from build123d import *

# Parameters (mm, degrees)
F0_R     = 10.8555352801
F1_DEPTH = 13
F2_T     = -2.5
F3_R     = 3.906627993
F4_DEPTH = 11.4
F5_T     = -1
F6_W     = 5.8806912699
F6_H     = 0.9425205584
F7_DEPTH = 12.4


with BuildPart() as f1:
    # F0 (on Top) → F1 (new body)
    with BuildSketch(Plane.XY):
        Circle(F0_R)
    extrude(amount=F1_DEPTH)

    # F2
    f2_openings = [f1.faces().sort_by_distance(p)[0] for p in [
        (0, 0, 0),
    ]]
    offset(amount=F2_T, openings=f2_openings)

    # F3 (on face) → F4 (join)
    with BuildSketch(Plane.XY.offset(13)):
        Circle(F3_R)
    extrude(amount=F4_DEPTH)

    # F5
    f5_openings = [f1.faces().sort_by_distance(p)[0] for p in [
        (0, 0, 24.4),
    ]]
    offset(amount=F5_T, openings=f5_openings, kind=Kind.INTERSECTION)

    # F6 (on face) → F7 (join)
    with BuildSketch(Plane.XY.offset(24.4)):
        with Locations((0.0686239588, 2.1773161103)):
            Rectangle(F6_W, F6_H)
    extrude(amount=-F7_DEPTH)


solid = f1.part
Check sheet for the modelled part. Datum: model origin and axes. Units: mm. A direction names the side the tool comes from. Coordinates: 2 decimals unless noted, no trailing zeros. Loops run counter-clockwise (first coordinate to the right, second up) from the corner with the lowest first, then second, coordinate; pieces in that order, holes last. Notation, with made-up numbers: (45, 48.25) -> (83, 48.25) arc R22 cw to (83, 73.25) -> close; hole circle Ø10 at (-13, 75.25). An arc over 180 degrees is marked (long way). Answer in a Markdown table with one row per item.
1. Sectioned sample at D-D, the plane y = -5. Record the boundary of the cut face in (x, z), then the cut area to 3 significant figures.
Check values:
| item | result |
|---|---|
| outline | (-9.64, 0) -> (-6.69, 0) -> (-6.69, 10.5) -> (6.69, 10.5) -> (6.69, 0) -> (9.64, 0) -> (9.64, 13) -> (-9.64, 13) -> close; hole (-8.49, 1) -> (-7.91, 1) -> (-7.91, 11.5) -> (7.91, 11.5) -> (7.91, 1) -> (8.49, 1) -> (8.49, 12) -> (-8.49, 12) -> close |
| area | 89.1 mm2 |
2. Sectioned sample at B-B, the plane x = 0. Record the boundary of the cut face in (y, z).
Check values:
| item | result |
|---|---|
| outline | (-10.86, 0) -> (-8.36, 0) -> (-8.36, 10.5) -> (8.36, 10.5) -> (8.36, 0) -> (10.86, 0) -> (10.86, 13) -> (3.91, 13) -> (3.91, 24.4) -> (2.91, 24.4) -> (2.91, 12) -> (9.86, 12) -> (9.86, 1) -> (9.36, 1) -> (9.36, 11.5) -> (-9.36, 11.5) -> (-9.36, 1) -> (-9.86, 1) -> (-9.86, 12) -> (-2.91, 12) -> (-2.91, 24.4) -> (-3.91, 24.4) -> (-3.91, 13) -> (-10.86, 13) -> close; (1.71, 12) -> (2.65, 12) -> (2.65, 24.4) -> (1.71, 24.4) -> close |
3. Material ranges on line 1 along Y through (x, z) = (0, 9.25); line 2 along Z through (x, y) = (0.25, 2); line 3 along Z through (x, y) = (-5, -8), recorded low to high. Write a range as [from, to].
Check values:
| item | result |
|---|---|
| line 1 | y = [-10.86, -9.86], [-9.36, -8.36], [8.36, 9.36], [9.86, 10.86] |
| line 2 | z = [10.5, 11.5], [12, 24.4] |
| line 3 | z = [0, 1], [12, 13] |
4. Release check for a two-part mould opening along Y. For faces 1 (the face through (0, 2, 24.4)), 2 (the face through (10.354, 3.261, 6.409)), 3 (the face through (0, 2, 12)) record: released by +Y, released by -Y, zero draft, split by the parting line, or undercut.
Check values:
| item | result |
|---|---|
| face 1 | zero draft |
| face 2 | split by the parting line |
| face 3 | undercut |
5. Go/stop test with flat-tipped pins: pin 1 (3 mm diameter, centred on y = 1.5, z = 13.5, fed in from +X); pin 2 (8.5 mm diameter, centred on x = 2.5, y = -2, fed in from -Z); pin 3 (8 mm diameter, centred on x = -8, z = 11.5, fed in from -Y); pin 4 (1.5 mm diameter, centred on x = -1, z = 6, fed in from +Y). Record where each tip stops, or that it passes through.
Check values:
| item | result |
|---|---|
| pin 1 | stops at x = 10.86 |
| pin 2 | stops at z = 10.5 |
| pin 3 | stops at y = -10.09 |
| pin 4 | stops at y = 10.85 |
6. Sectioned sample at C-C, the plane z = 8.5. Record the boundary of the cut face in (x, y), then the cut area to 3 significant figures.
Check values:
| item | result |
|---|---|
| outline | circle Ø21.71 at (0, 0); circle Ø18.71 at (0, 0); hole circle Ø19.71 at (0, 0); hole circle Ø16.71 at (0, 0) |
| area | 121 mm2 |
7. Sectioned sample at A-A, the plane z = 20.25. Record the boundary of the cut face in (x, y), then the cut area to 3 significant figures.
Check values:
| item | result |
|---|---|
| outline | (2.87, 2.65) arc R3.91 ccw (long way) to (3.01, 2.49) -> (3.01, 2.65) -> close; hole (-2.35, 1.71) arc R2.91 ccw (long way) to (2.35, 1.71) -> close; hole (-1.2, 2.65) -> (1.2, 2.65) arc R2.91 ccw to start |
| area | 25.0 mm2 |
8. Access from +Z, -Z, +X, -X, +Y, -Y to the whole of each face (thin tool, end or side, straight path). Record for faces 4 (the face through (7.97, 2.51, 5.18)), 5 (the face through (0, 1.706, 18)), 6 (the face through (0, 0, 11.5)).
Check values:
| item | result |
|---|---|
| face 4 | -Z |
| face 5 | +Z |
| face 6 | none |
